```python
from build123d import *

# Parameters (mm, degrees)
SKETCH1_R      = 0.75
EXTRUDE1_DEPTH = 0.81
CHAMFER4_SIZE  = 1
CHAMFER4_SIZE2 = 0.176326981
CHAMFER5_SIZE  = 1
CHAMFER5_SIZE2 = 0.176326981
CHAMFER1_SIZE  = 1
SKETCH2_W      = 0.762
SKETCH2_H      = 0.81
EXTRUDE2_DEPTH = 1.14
SKETCH3_W      = 0.762
SKETCH3_H      = 0.81
EXTRUDE3_DEPTH = 1.14
FILLET1_R      = 0.5
FILLET2_R      = 1.31


with BuildPart() as part:
    # Sketch1 → Extrude1 (new body)
    with BuildSketch(Plane.XY):
        with BuildLine():
            Line((-3.175, 4.52), (3.175, 4.52))
            Line((3.175, 4.52), (3.175, -3.4))
            Line((3.175, -3.4), (3.96, -3.4))
            Line((3.96, -3.4), (3.96, -5.69))
            Line((3.96, -5.69), (3.175, -5.69))
            Line((3.175, -5.69), (3.175, -7.595))
            Line((3.175, -7.595), (2.921867651, -9.286989911))
            ThreePointArc((2.921867651, -9.286989911), (2.837794855, -9.43940364), (2.674619301, -9.5))
            Line((2.674619301, -9.5), (2.405380699, -9.5))
            ThreePointArc((2.405380699, -9.5), (2.242205145, -9.43940364), (2.158132349, -9.286989911))
            Line((2.158132349, -9.286989911), (1.905, -7.595))
            Line((1.905, -7.595), (1.905, -4.225996329))
            ThreePointArc((1.905, -4.225996329), (1.676788936, -3.976947655), (1.408798062, -4.182584285))
            Line((1.408798062, -4.182584285), (1.143, -5.69))
            Line((1.143, -5.69), (0.381, -5.69))
            Line((0.381, -5.69), (0.249019923, -4.203881227))
            ThreePointArc((0.249019923, -4.203881227), (0, -3.975996329), (-0.249019923, -4.203881227))
            Line((-0.249019923, -4.203881227), (-0.381, -5.69))
            Line((-0.381, -5.69), (-1.143, -5.69))
            Line((-1.143, -5.69), (-1.408798062, -4.182584285))
            ThreePointArc((-1.408798062, -4.182584285), (-1.676788936, -3.976947655), (-1.905, -4.225996329))
            Line((-1.905, -4.225996329), (-1.905, -7.595))
            Line((-1.905, -7.595), (-2.158132349, -9.286989911))
            ThreePointArc((-2.158132349, -9.286989911), (-2.242205145, -9.43940364), (-2.405380699, -9.5))
            Line((-2.405380699, -9.5), (-2.674619301, -9.5))
            ThreePointArc((-2.674619301, -9.5), (-2.837794855, -9.43940364), (-2.921867651, -9.286989911))
            Line((-2.921867651, -9.286989911), (-3.175, -7.595))
            Line((-3.175, -7.595), (-3.175, -5.69))
            Line((-3.175, -5.69), (-3.96, -5.69))
            Line((-3.96, -5.69), (-3.96, -3.4))
            Line((-3.96, -3.4), (-3.175, -3.4))
            Line((-3.175, -3.4), (-3.175, 4.52))
        make_face()
        Circle(SKETCH1_R, mode=Mode.SUBTRACT)
    extrude(amount=EXTRUDE1_DEPTH)

    # Chamfer4
    chamfer4_edges = [part.edges().sort_by_distance(p)[0] for p in [
        (0, 4.52, 0.81),
    ]]
    chamfer4_side = [part.faces().sort_by_distance(p)[0] for p in [
        (0, -1.422995991, 0.81),
    ]]
    chamfer(chamfer4_edges, length=CHAMFER4_SIZE, length2=CHAMFER4_SIZE2, reference=chamfer4_side[0])

    # Chamfer5
    chamfer5_edges = [part.edges().sort_by_distance(p)[0] for p in [
        (0, 4.52, 0),
    ]]
    chamfer5_side = [part.faces().sort_by_distance(p)[0] for p in [
        (0, -1.422995991, 0),
    ]]
    chamfer(chamfer5_edges, length=CHAMFER5_SIZE, length2=CHAMFER5_SIZE2, reference=chamfer5_side[0])

    # Chamfer1
    chamfer1_edges = [part.edges().sort_by_distance(p)[0] for p in [
        (-3.175, 4.52, 0.405),
        (3.175, 4.52, 0.405),
    ]]
    chamfer(chamfer1_edges, length=CHAMFER1_SIZE)

    # Sketch2 → Extrude2 (add)
    with BuildSketch(Plane.XY.offset(0.81)):
        with Locations((-0.762, -5.285)):
            Rectangle(SKETCH2_W, SKETCH2_H)
    extrude(amount=EXTRUDE2_DEPTH)

    # Sketch3 → Extrude3 (add)
    with BuildSketch(Plane(origin=(0, 0, 0), x_dir=(-1, 0, 0), z_dir=(0, 0, -1))):
        with Locations((-0.762, -5.285)):
            Rectangle(SKETCH3_W, SKETCH3_H)
    extrude(amount=EXTRUDE3_DEPTH)

    # Fillet1
    fillet1_edges = [part.edges().sort_by_distance(p)[0] for p in [
        (-0.762, -4.88, 0.81),
        (0.762, -4.88, 0),
    ]]
    fillet(fillet1_edges, radius=FILLET1_R)

    # Fillet2
    # the kernel refuses this fillet: 1.31 mm, written as the material it takes off along each edge
    with BuildSketch(Plane(origin=(2.894, -5.69, 0), x_dir=(0, 1, 0), z_dir=(-1, 0, 0))) as fillet2_piece_1_section:
        with BuildLine():
            CenterArc((FILLET2_R, -FILLET2_R), FILLET2_R, 90, 90)
            Line((0, -FILLET2_R), (0, 0))
            Line((0, 0), (FILLET2_R, 0))
        make_face()
    fillet2_piece_1 = extrude(amount=7.312, mode=Mode.PRIVATE)
    fillet2_piece_1 = split(fillet2_piece_1, bisect_by=Plane(origin=(-1.183630383, -5.45957365, 0.262964563), z_dir=(0.984807753012208, 0.17364817766693083, 0)), keep=Keep.TOP, mode=Mode.PRIVATE)
    fillet2_piece_1 = split(fillet2_piece_1, bisect_by=Plane(origin=(0.345201257, -5.286899882, 0.262964563), z_dir=(-0.9960796936325239, -0.08846040884450787, 0)), keep=Keep.TOP, mode=Mode.PRIVATE)
    add(fillet2_piece_1, mode=Mode.SUBTRACT)
    with BuildSketch(Plane(origin=(4.418, -5.69, 0.81), x_dir=(0, 1, 0), z_dir=(-1, 0, 0))) as fillet2_piece_2_section:
        with BuildLine():
            CenterArc((FILLET2_R, FILLET2_R), FILLET2_R, 180, 90)
            Line((0, FILLET2_R), (0, 0))
            Line((0, 0), (FILLET2_R, 0))
        make_face()
    fillet2_piece_2 = extrude(amount=7.312, mode=Mode.PRIVATE)
    fillet2_piece_2 = split(fillet2_piece_2, bisect_by=Plane(origin=(1.905, -5.189166234, 0.641921168), z_dir=(-1, 0, 0)), keep=Keep.TOP, mode=Mode.PRIVATE)
    fillet2_piece_2 = split(fillet2_piece_2, bisect_by=Plane(origin=(0.343178087, -5.264118635, 0.641921168), z_dir=(0.9960796936325239, 0.08846040884450787, 0)), keep=Keep.TOP, mode=Mode.PRIVATE)
    add(fillet2_piece_2, mode=Mode.SUBTRACT)


solid = part.part
```
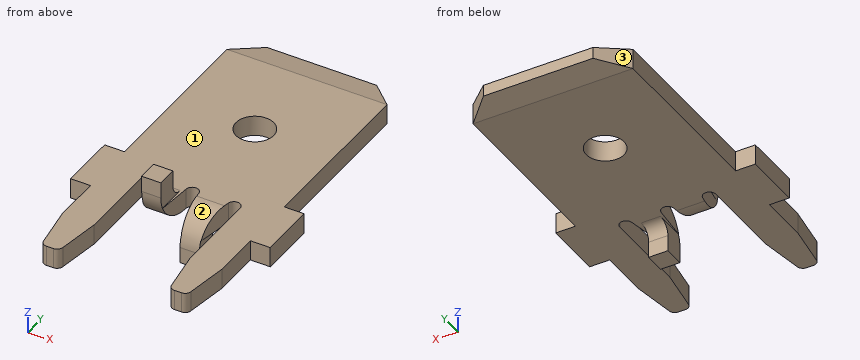
Can you work these out from the model? Positions are in its coordinate system, mm. Face numbers are marked on the shaded views. Coordinates: 2 decimals unless noted, no trailing zeros. Loops run counter-clockwise (first coordinate to the right, second up) from the corner with the lowest first, then second, coordinate; pieces in that order, holes last. Notation, with made-up numbers: M 60.25,11.25 L 70.25,11.25 A24 cw 70.25,43.25 Z; hole C 89.5,-0.75 d1. An arc over 180 degrees is marked long. Put each result on its own line as item: value. Start each with the question number.
(1) Imagine slicing it at A-A on x = 0. List the corners of the cut face in (y, z) for me, and give its area (3 significant figures).
(2) Will these pins go through, and if not, where does the flat tip stop? pin 1 Ø0.5 at (x, z) = (0.5, -1) entering from +Y; pin 2 Ø1.3 at (y, z) = (-5.5, 1.5) entering from +X; pin 3 Ø4 at (x, y) = (-2, -4.5) entering from -Z; pin 4 Ø0.9 at (x, y) = (0, 0) entering from +Z.
(3) I need wall thicknesses on probe 1 along Y at (x, z) = (0, 0.6); probe 2 along Z at (x, y) = (0.25, 1.5); probe 3 along X at (y, z) = (1, 0.25) (3 decimals). Which ranges of each line are inside material? Lowest first, please.
(4) Imagine slicing it at D-D on x = 1. List the corners of the cut face in (y, z) for me, and give its area (3 significant figures).
(5) Imagine slicing it at B-B on y = 0. List the corners of the cut face in (x, z) for me (3 decimals).
(6) We'd pull the mould along X, two halves only. Please class the marked faces 1, 2 and 3: +X half, -X half, draft (parallel to the pull), parting line (faces both ways), or undercut.
(7) Imagine slicing it at C-C on y = -6.5. List the corners of the cut face in (x, z) for me (3 decimals).
Worked answers:
1. outline: M -3.98,0 L -0.75,0 L -0.75,0.81 L -3.98,0.81 Z; M 0.75,0 L 3.52,0 L 4.52,0.18 L 4.52,0.63 L 3.52,0.81 L 0.75,0.81 Z
1. area: 5.49 mm2
2. pin 1: stops at y = -4.88
2. pin 2: stops at x = -0.38
2. pin 3: stops at z = 0
2. pin 4: passes through
3. probe 1: y = -3.98 to -0.75, 0.75 to 4.52
3. probe 2: z = 0 to 0.81
3. probe 3: x = -3.175 to 3.175
4. outline: M -5.69,-1.14 L -4.88,-1.14 L -4.88,-0.5 A0.5 cw -4.38,0 L 3.52,0 L 4.52,0.18 L 4.52,0.63 L 3.52,0.81 L -4.38,0.81 A1.31 ccw -5.69,-0.5 Z
4. area: 8.70 mm2
5. outline: M -3.175,0 L -0.75,0 L -0.75,0.81 L -3.175,0.81 Z; M 0.75,0 L 3.175,0 L 3.175,0.81 L 0.75,0.81 Z
6. face 1: draft
6. face 2: undercut
6. face 3: -X half
7. outline: M -3.175,0 L -1.905,0 L -1.905,0.81 L -3.175,0.81 Z; M 1.905,0 L 3.175,0 L 3.175,0.81 L 1.905,0.81 Z
